The listing builds one solid part. Answer for the finished solid, in the listing's coordinates (mm). A direction names the side the tool comes from. Round coordinates to 2 decimals unless told otherwise and drop trailing zeros. Write each loop counter-clockwise with the first axis right and the second up, starting at its lowest first coordinate (ties: lowest second). Pieces come first, ordered by that corner, then holes. Notation, with made-up numbers: M -5,-39 L 34,-39 A14 cw 34,-14 Z; hole C 83.5,13 d1. An arc over 180 degrees is marked long. One line per item, written item: value. Start each with the question number.
(1) For faces 4 (the flat face through (180, 63.5, 6)), 5 (the cylindrical face through (76.203, 31.471, 6.261)), determine the directions among +Z, -Z, +X, -X, +Y, -Y from which every point of the face is accessible in a straight line to the end or side of a thin tool.
(2) Section B-B (z = 4) is taken. Determine the outline of the cut face in (x, y), plus the area to 3 significant figures.
(3) Section A-A (x = 173) is taken. Determine the outline of the cut face in (y, z).
(4) For a pull along X with two mould halves and no side action, classify faces 1 (the flat face through (179, 44.45, 6)), 2 (the flat face through (0, 32, 6)), 3 (the flat face through (175, 46, 0)) as released by +X, released by -X, zero draft, split by the parting line, or undercut.
(5) Consider probe 1 along Y at (x, z) = (242, 3); probe 2 along X at (y, z) = (34, 9.25); probe 3 along X at (y, z) = (28.5, 6.5). Determine where each line is inside the solid, lowest interval first.
(6) Section C-C (y = 31.75) is taken. Determine the outline of the cut face in (x, z).
Autodesk Inventor part; units mm, degrees
ref_plane "YZ Plane" through (0, 0, 0) normal (1, 0, 0) x (0, 1, 0)
ref_plane "XZ Plane" through (0, 0, 0) normal (0, 1, 0) x (-1, 0, 0)
ref_plane "XY Plane" through (0, 0, 0) normal (0, 0, 1) x (1, 0, 0)
sketch "Sketch1" plane through (0, 0, 0) normal (0, 0, 1) x (1, 0, 0)
  line L0 (0, 0) -> (355.6, 0)
  line L1 (355.6, 0) -> (355.6, 63.5)
  line L2 (355.6, 63.5) -> (0, 63.5)
  line L3 (0, 63.5) -> (0, 0)
  line L4 (88.9, 31.75) -> (266.7, 31.75) construction
  line L5 (88.9, 19.05) -> (266.7, 19.05)
  line L6 (266.7, 44.45) -> (88.9, 44.45)
  arc A0 (88.9, 44.45) -> (88.9, 19.05) centre (88.9, 31.75) ccw
  arc A1 (266.7, 19.05) -> (266.7, 44.45) centre (266.7, 31.75) ccw
  point P0 (177.8, 31.75)
  dimension "d0" = 355.6
  dimension "d1" = 63.5
  dimension "d4" = 25.4
  dimension "d5" = 177.8
  dimension "d6" = 177.8
extrude "Extrusion1" add sketch "Sketch1" along normal blind 12.7
properties part number "Electronics Side Plate"
Recorded:
1. face 4: +Z, -Z, +X, -X, +Y
1. face 5: +Z, -Z
2. outline: M 0,0 L 355.6,0 L 355.6,63.5 L 0,63.5 Z; hole M 88.9,19.05 L 266.7,19.05 A12.7 ccw 266.7,44.45 L 88.9,44.45 A12.7 ccw Z
2. area: 17,600 mm2
3. outline: M 0,0 L 19.05,0 L 19.05,12.7 L 0,12.7 Z; M 44.45,0 L 63.5,0 L 63.5,12.7 L 44.45,12.7 Z
4. face 1: undercut
4. face 2: released by -X
4. face 3: zero draft
5. probe 1: y = 0 to 19.05, 44.45 to 63.5
5. probe 2: x = 0 to 76.4, 279.2 to 355.6
5. probe 3: x = 0 to 76.62, 278.98 to 355.6
6. outline: M 0,0 L 76.2,0 L 76.2,12.7 L 0,12.7 Z; M 279.4,0 L 355.6,0 L 355.6,12.7 L 279.4,12.7 Z
